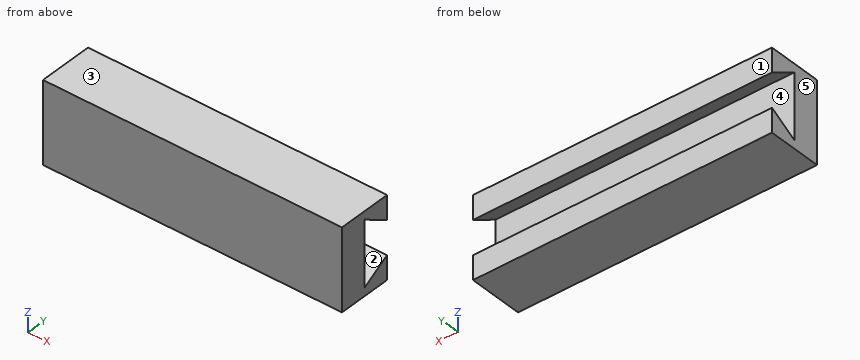
Autodesk Inventor part; units mm, degrees
ref_plane "YZ Plane" through (0, 0, 0) normal (1, 0, 0) x (0, 1, 0)
ref_plane "XZ Plane" through (0, 0, 0) normal (0, 1, 0) x (-1, 0, 0)
ref_plane "XY Plane" through (0, 0, 0) normal (0, 0, 1) x (1, 0, 0)
sketch "Sketch4" plane through (0, 0, 0) normal (1, 0, 0) x (0, 1, 0)
  line L0 (0, 0) -> (0, -12)
  line L1 (0, -12) -> (10, -6.2265)
  line L2 (10, -6.2265) -> (10, 6.2265) construction
  line L3 (10, 6.2265) -> (0, 12)
  line L4 (0, 12) -> (0, 0)
  line L5 (0, 0) -> (10, 0) construction
  line L6 (10, 6.2265) -> (10, 15)
  line L7 (10, 15) -> (-10, 15)
  line L8 (-10, 15) -> (-10, -15)
  line L9 (-10, -15) -> (10, -15)
  line L10 (10, -15) -> (10, -6.2265)
  dimension "d31" = 60
  dimension "d32" = 60
  dimension "d33" = 10
  dimension "d34" = 12
  dimension "d43" = 10
  dimension "d44" = 30
extrude "Extrusion3" add sketch "Sketch4" along normal mid plane 110
properties part number "Runway" material "Acero, carbono"
Geometry: final body of the model. Coordinates: model frame, mm. Face numbers are marked on the shaded views. A direction names the side the tool comes from. Coordinates: 2 decimals unless noted, no trailing zeros. Order: outer loops, then holes, each group sorted by start corner. A loop starts at its lowest first (then second) coordinate and runs counter-clockwise, first axis right, second up.
1) Section D-D (z = 4.75). Return loops of the section in (x, y), then the cut area to 3 significant figures.
Result sheet:
outline: (-55, -10) - (55, -10) - (55, 0) - (-55, 0) - close
area: 1,100 mm2
2) Section B-B (z = 9). Return loops of the section in (x, y).
Result sheet:
outline: (-55, -10) - (55, -10) - (55, 0) - (-55, 0) - close; (-55, 5.2) - (55, 5.2) - (55, 10) - (-55, 10) - close
3) Set-up query: the marked faces 4 and 5. Return all of +Z, -Z, +X, -X, +Y, -Y with unobstructed straight access to the full face (end or side cutting, diameter ignored); none if empty.
Result sheet:
face 4: +X, -X
face 5: +Z, -Z, -X, +Y, -Y
4) Section A-A (x = -21). Return loops of the section in (y, z), then the cut area to 3 significant figures.
Result sheet:
outline: (-10, -15) - (10, -15) - (10, -6.23) - (0, -12) - (0, 12) - (10, 6.23) - (10, 15) - (-10, 15) - close
area: 418 mm2
5) Section C-C (y = 3). Return loops of the section in (x, z), then the cut area to 3 significant figures.
Result sheet:
outline: (-55, -15) - (55, -15) - (55, -10.27) - (-55, -10.27) - close; (-55, 10.27) - (55, 10.27) - (55, 15) - (-55, 15) - close
area: 1,040 mm2
6) Ray query, probe 1 along Y at (x, z) = (-11, 5.5); probe 2 along Z at (x, y) = (30.5, 0.5); probe 3 along Z at (x, y) = (21.5, 3.5). Return the intervals inside material, ascending.
Result sheet:
probe 1: y = -10 to 0
probe 2: z = -15 to -11.71, 11.71 to 15
probe 3: z = -15 to -9.98, 9.98 to 15
7) Draft query along Y for the marked faces 1, 2 and 3. Return one class per face: released by +Y, released by -Y, zero draft, split by the parting line, or undercut.
Result sheet:
face 1: released by +Y
face 2: undercut
face 3: zero draft
